```python
from build123d import *

# Parameters (mm, degrees)
SKETCH_1_W          = 20
SKETCH_1_H          = 20
EXTRUDE_1_DEPTH     = 182
SKETCH_3_W          = 35
SKETCH_3_H          = 35
EXTRUDE_2_DEPTH     = 3
SKETCH_4_R          = 2.1
CUT_EXTRUDE_2_DEPTH = 23
CUT_EXTRUDE_3_REACH = 188.648
SKETCH_5_R          = 1.6
EXTRUDE_3_DEPTH     = 20
EXTRUDE_4_DEPTH     = 20
FILLET_1_R          = 2
CUT_EXTRUDE_4_REACH = 186.903
SKETCH_8_W          = 62
SKETCH_8_H          = 12
CUT_EXTRUDE_6_REACH = 186.896


with BuildPart() as part:
    # 草图1 → 凸台-拉伸1 (new body)
    with BuildSketch(Plane(origin=(0, 0, 0), x_dir=(0, 0, -1), z_dir=(1, 0, 0))):
        Rectangle(SKETCH_1_W, SKETCH_1_H)
    extrude(amount=EXTRUDE_1_DEPTH)

    # 草图3 → 凸台-拉伸2 (add)
    with BuildSketch(Plane.ZY):
        Rectangle(SKETCH_3_W, SKETCH_3_H)
    extrude(amount=EXTRUDE_2_DEPTH)

    # 草图4 → 切除-拉伸2 (cut)
    with BuildSketch(Plane(origin=(182, 0, 0), x_dir=(0, 0, -1), z_dir=(1, 0, 0))):
        Circle(SKETCH_4_R)
    extrude(amount=-CUT_EXTRUDE_2_DEPTH, mode=Mode.SUBTRACT)

    # 草图5 → 切除-拉伸3 (cut, up to next)
    with BuildSketch(Plane.ZY.offset(3), mode=Mode.PRIVATE) as cut_extrude_3_sk1:
        with Locations((-14, 14)):
            Circle(SKETCH_5_R)
    cut_extrude_3_tool1 = extrude(cut_extrude_3_sk1.sketch, amount=-CUT_EXTRUDE_3_REACH, mode=Mode.PRIVATE) & part.part
    # 草图5 → 切除-拉伸3 (cut, up to next)
    with BuildSketch(Plane.ZY.offset(3), mode=Mode.PRIVATE) as cut_extrude_3_sk2:
        with Locations((14, 14)):
            Circle(SKETCH_5_R)
    cut_extrude_3_tool2 = extrude(cut_extrude_3_sk2.sketch, amount=-CUT_EXTRUDE_3_REACH, mode=Mode.PRIVATE) & part.part
    # 草图5 → 切除-拉伸3 (cut, up to next)
    with BuildSketch(Plane.ZY.offset(3), mode=Mode.PRIVATE) as cut_extrude_3_sk3:
        with Locations((-14, -14)):
            Circle(SKETCH_5_R)
    cut_extrude_3_tool3 = extrude(cut_extrude_3_sk3.sketch, amount=-CUT_EXTRUDE_3_REACH, mode=Mode.PRIVATE) & part.part
    # 草图5 → 切除-拉伸3 (cut, up to next)
    with BuildSketch(Plane.ZY.offset(3), mode=Mode.PRIVATE) as cut_extrude_3_sk4:
        with Locations((14, -14)):
            Circle(SKETCH_5_R)
    cut_extrude_3_tool4 = extrude(cut_extrude_3_sk4.sketch, amount=-CUT_EXTRUDE_3_REACH, mode=Mode.PRIVATE) & part.part
    add(cut_extrude_3_tool1.solids().sort_by_distance((-3, 14, -14))[0], mode=Mode.SUBTRACT)
    add(cut_extrude_3_tool2.solids().sort_by_distance((-3, 14, 14))[0], mode=Mode.SUBTRACT)
    add(cut_extrude_3_tool3.solids().sort_by_distance((-3, -14, -14))[0], mode=Mode.SUBTRACT)
    add(cut_extrude_3_tool4.solids().sort_by_distance((-3, -14, 14))[0], mode=Mode.SUBTRACT)

    # 草图6 → 凸台-拉伸3 (add)
    with BuildSketch(Plane(origin=(0, 0, -10), x_dir=(-1, 0, 0), z_dir=(0, 0, -1))):
        Polygon((-30, 10), (0, 17.5), (0, 10), align=None)
        Polygon((0, -10), (-30, -10), (0, -17.5), align=None)
    extrude(amount=-EXTRUDE_3_DEPTH)

    # 草图7 → 凸台-拉伸4 (add)
    with BuildSketch(Plane(origin=(0, 10, 0), x_dir=(1, 0, 0), z_dir=(0, 1, 0))):
        Polygon((0, 10), (30, 10), (0, 17.5), align=None)
        Polygon((30, -10), (0, -10), (0, -17.550639808), align=None)
    extrude(amount=-EXTRUDE_4_DEPTH)

    # 圆角1
    # the kernel refuses this fillet: 2 mm, written as the material it adds along each edge
    with BuildSketch(Plane(origin=(-5, 10, -10), x_dir=(0, 0, -1), z_dir=(1, 0, 0))) as fillet_1_piece_1_section:
        with BuildLine():
            CenterArc((FILLET_1_R, FILLET_1_R), FILLET_1_R, 180, 90)
            Line((0, FILLET_1_R), (0, 0))
            Line((0, 0), (FILLET_1_R, 0))
        make_face()
    fillet_1_piece_1 = extrude(amount=40, mode=Mode.PRIVATE)
    fillet_1_piece_1 = split(fillet_1_piece_1, bisect_by=Plane(origin=(14.470095562, 13.882476109, -10.438694278), z_dir=(-0.24253562503633314, -0.9701425001453319, 0)), keep=Keep.TOP, mode=Mode.PRIVATE)
    fillet_1_piece_1 = split(fillet_1_piece_1, bisect_by=Plane(origin=(-3, 10.438694278, -10.438694278), z_dir=(1, 0, 0)), keep=Keep.TOP, mode=Mode.PRIVATE)
    fillet_1_piece_1 = split(fillet_1_piece_1, bisect_by=Plane(origin=(14.470095562, 10.438694278, -13.882476109), z_dir=(-0.24253562503633308, 0, 0.9701425001453319)), keep=Keep.TOP, mode=Mode.PRIVATE)
    add(fillet_1_piece_1)
    with BuildSketch(Plane(origin=(0, -10, -10), x_dir=(0, -1, 0), z_dir=(1, 0, 0))) as fillet_1_piece_2_section:
        with BuildLine():
            CenterArc((FILLET_1_R, FILLET_1_R), FILLET_1_R, 180, 90)
            Line((0, FILLET_1_R), (0, 0))
            Line((0, 0), (FILLET_1_R, 0))
        make_face()
    fillet_1_piece_2 = extrude(amount=35, mode=Mode.PRIVATE)
    fillet_1_piece_2 = split(fillet_1_piece_2, bisect_by=Plane(origin=(14.470095562, -10.438694278, -13.882476109), z_dir=(-0.24253562503633308, 0, 0.9701425001453319)), keep=Keep.TOP, mode=Mode.PRIVATE)
    fillet_1_piece_2 = split(fillet_1_piece_2, bisect_by=Plane(origin=(14.470095562, -13.882476109, -10.438694278), z_dir=(-0.24253562503633314, 0.9701425001453319, 0)), keep=Keep.TOP, mode=Mode.PRIVATE)
    add(fillet_1_piece_2)
    with BuildSketch(Plane(origin=(35, 10, 10), x_dir=(0, 1, 0), z_dir=(-1, 0, 0))) as fillet_1_piece_3_section:
        with BuildLine():
            CenterArc((FILLET_1_R, -FILLET_1_R), FILLET_1_R, 90, 90)
            Line((0, -FILLET_1_R), (0, 0))
            Line((0, 0), (FILLET_1_R, 0))
        make_face()
    fillet_1_piece_3 = extrude(amount=40, mode=Mode.PRIVATE)
    fillet_1_piece_3 = split(fillet_1_piece_3, bisect_by=Plane(origin=(14.474382617, 13.881404346, 10.438850692), z_dir=(-0.24253562503633314, -0.9701425001453319, 0)), keep=Keep.TOP, mode=Mode.PRIVATE)
    fillet_1_piece_3 = split(fillet_1_piece_3, bisect_by=Plane(origin=(-3, 10.438597443, 10.438850692), z_dir=(1, 0, 0)), keep=Keep.TOP, mode=Mode.PRIVATE)
    fillet_1_piece_3 = split(fillet_1_piece_3, bisect_by=Plane(origin=(14.485990983, 10.438597443, 13.904689802), z_dir=(-0.24407597060240918, 0, -0.969756113966028)), keep=Keep.TOP, mode=Mode.PRIVATE)
    add(fillet_1_piece_3)
    with BuildSketch(Plane(origin=(35, -10, 10), x_dir=(0, 0, 1), z_dir=(-1, 0, 0))) as fillet_1_piece_4_section:
        with BuildLine():
            CenterArc((FILLET_1_R, -FILLET_1_R), FILLET_1_R, 90, 90)
            Line((0, -FILLET_1_R), (0, 0))
            Line((0, 0), (FILLET_1_R, 0))
        make_face()
    fillet_1_piece_4 = extrude(amount=35, mode=Mode.PRIVATE)
    fillet_1_piece_4 = split(fillet_1_piece_4, bisect_by=Plane(origin=(14.474382617, -13.881404346, 10.438850692), z_dir=(-0.24253562503633314, 0.9701425001453319, 0)), keep=Keep.TOP, mode=Mode.PRIVATE)
    fillet_1_piece_4 = split(fillet_1_piece_4, bisect_by=Plane(origin=(14.485990983, -10.438597443, 13.904689802), z_dir=(-0.24407597060240918, 0, -0.969756113966028)), keep=Keep.TOP, mode=Mode.PRIVATE)
    add(fillet_1_piece_4)

    # 草图8 → 切除-拉伸4 (cut, up to next)
    with BuildSketch(Plane(origin=(0, 0, -10), x_dir=(-1, 0, 0), z_dir=(0, 0, -1)), mode=Mode.PRIVATE) as cut_extrude_4_sk1:
        with Locations((-147, 0)):
            Rectangle(SKETCH_8_W, SKETCH_8_H)
    cut_extrude_4_tool1 = extrude(cut_extrude_4_sk1.sketch, amount=-CUT_EXTRUDE_4_REACH, mode=Mode.PRIVATE) & part.part
    add(cut_extrude_4_tool1.solids().sort_by_distance((147, 0, -10))[0], mode=Mode.SUBTRACT)

    # 草图9 → 切除-拉伸6 (cut, up to next)
    with BuildSketch(Plane.XY.offset(10), mode=Mode.PRIVATE) as cut_extrude_6_sk1:
        with BuildLine():
            Line((97.964235065, 6.297490727), (107.103469291, -2.781172596))
            ThreePointArc((107.103469291, -2.781172596), (107.115824812, -6.497340056), (103.399657352, -6.509695577))
            Line((103.399657352, -6.509695577), (94.260423126, 2.568967746))
            ThreePointArc((94.260423126, 2.568967746), (94.248067605, 6.285135206), (97.964235065, 6.297490727))
        make_face()
    cut_extrude_6_tool1 = extrude(cut_extrude_6_sk1.sketch, amount=-CUT_EXTRUDE_6_REACH, mode=Mode.PRIVATE) & part.part
    # 草图9 → 切除-拉伸6 (cut, up to next)
    with BuildSketch(Plane.XY.offset(10), mode=Mode.PRIVATE) as cut_extrude_6_sk2:
        with BuildLine():
            Line((82.964235065, 6.297490727), (92.103469291, -2.781172596))
            ThreePointArc((92.103469291, -2.781172596), (92.115824812, -6.497340056), (88.399657352, -6.509695577))
            Line((88.399657352, -6.509695577), (79.260423126, 2.568967746))
            ThreePointArc((79.260423126, 2.568967746), (79.248067605, 6.285135206), (82.964235065, 6.297490727))
        make_face()
    cut_extrude_6_tool2 = extrude(cut_extrude_6_sk2.sketch, amount=-CUT_EXTRUDE_6_REACH, mode=Mode.PRIVATE) & part.part
    # 草图9 → 切除-拉伸6 (cut, up to next)
    with BuildSketch(Plane.XY.offset(10), mode=Mode.PRIVATE) as cut_extrude_6_sk3:
        with BuildLine():
            Line((67.964235065, 6.297490727), (77.103469291, -2.781172596))
            ThreePointArc((77.103469291, -2.781172596), (77.115824812, -6.497340056), (73.399657352, -6.509695577))
            Line((73.399657352, -6.509695577), (64.260423126, 2.568967746))
            ThreePointArc((64.260423126, 2.568967746), (64.248067605, 6.285135206), (67.964235065, 6.297490727))
        make_face()
    cut_extrude_6_tool3 = extrude(cut_extrude_6_sk3.sketch, amount=-CUT_EXTRUDE_6_REACH, mode=Mode.PRIVATE) & part.part
    # 草图9 → 切除-拉伸6 (cut, up to next)
    with BuildSketch(Plane.XY.offset(10), mode=Mode.PRIVATE) as cut_extrude_6_sk4:
        with BuildLine():
            Line((52.964235065, 6.297490727), (62.103469291, -2.781172596))
            ThreePointArc((62.103469291, -2.781172596), (62.115824812, -6.497340056), (58.399657352, -6.509695577))
            Line((58.399657352, -6.509695577), (49.260423126, 2.568967746))
            ThreePointArc((49.260423126, 2.568967746), (49.248067605, 6.285135206), (52.964235065, 6.297490727))
        make_face()
    cut_extrude_6_tool4 = extrude(cut_extrude_6_sk4.sketch, amount=-CUT_EXTRUDE_6_REACH, mode=Mode.PRIVATE) & part.part
    # 草图9 → 切除-拉伸6 (cut, up to next)
    with BuildSketch(Plane.XY.offset(10), mode=Mode.PRIVATE) as cut_extrude_6_sk5:
        with BuildLine():
            Line((37.964235065, 6.297490727), (47.103469291, -2.781172596))
            ThreePointArc((47.103469291, -2.781172596), (47.115824812, -6.497340056), (43.399657352, -6.509695577))
            Line((43.399657352, -6.509695577), (34.260423126, 2.568967746))
            ThreePointArc((34.260423126, 2.568967746), (34.248067605, 6.285135206), (37.964235065, 6.297490727))
        make_face()
    cut_extrude_6_tool5 = extrude(cut_extrude_6_sk5.sketch, amount=-CUT_EXTRUDE_6_REACH, mode=Mode.PRIVATE) & part.part
    add(cut_extrude_6_tool1.solids().sort_by_distance((100.681946, -0.106102, 10))[0], mode=Mode.SUBTRACT)
    add(cut_extrude_6_tool2.solids().sort_by_distance((85.681946, -0.106102, 10))[0], mode=Mode.SUBTRACT)
    add(cut_extrude_6_tool3.solids().sort_by_distance((70.681946, -0.106102, 10))[0], mode=Mode.SUBTRACT)
    add(cut_extrude_6_tool4.solids().sort_by_distance((55.681946, -0.106102, 10))[0], mode=Mode.SUBTRACT)
    add(cut_extrude_6_tool5.solids().sort_by_distance((40.681946, -0.106102, 10))[0], mode=Mode.SUBTRACT)


solid = part.part
```
Can you work these out from the model? Positions are in its coordinate system, mm. A direction names the side the tool comes from. Round coordinates to 2 decimals unless told otherwise and drop trailing zeros. Loops run counter-clockwise (first coordinate to the right, second up) from the corner with the lowest first, then second, coordinate; pieces in that order, holes last.
Item 1: Will these pins go through, and if not, where does the flat tip stop? pin 1 Ø1.5 at (x, z) = (157, -2.5) entering from -Y; pin 2 Ø4.5 at (x, z) = (10.5, -14) entering from +Y; pin 3 Ø5 at (x, y) = (65.5, 0.5) entering from +Z.
Item 2: Suppose I cut it at A-A, the plane x = 150. Write out the boundary of the cut face in (y, z), then the cut area to 3 significant figures.
Item 3: Suppose I cut it at C-C, the plane z = -5.5. State how many separate pieces and enclosed holes the cut face has, then the cut area to 3 significant figures.
Item 4: Suppose I cut it at B-B, the plane y = -14. Write out the boundary of the cut face in (x, z), then the cut area to 3 significant figures.
Item 5: Suppose I cut it at D-D, the plane z = 14. Write out the boundary of the cut face in (x, y).
Item 6: Which directions (+Z, -Z, +X, -X, +Y, -Y) give clear straight access to the entire face, cutting with the end or side of a thin tool? Please do faces 1 (the flat face through (0, 14, 12)), 2 (the flat face through (53.89, -2.03, 0.14)), 3 (the flat face through (0, -12, -14)).
Item 7: If we mould it in two halves opening along Y, with no side actions, what happens to faces 4 (the flat face through (8, -14, 10)), 5 (the flat face through (102.47, 1.82, 0.14)), 6 (the flat face through (105, 10, 0))? For each: +Y half, -Y half, draft (parallel to the pull), parting line (faces both ways), or undercut.
Item 8: Please list where these lines run through material, in increasing order: L1, parallel to Y at x = -1, z = -14; L2, parallel to Y at x = 142, z = 5.5; L3, parallel to Y at x = 179.05, z = 0.
Reported:
1. pin 1: stops at y = -10
1. pin 2: stops at y = 10.02
1. pin 3: stops at z = 10
2. outline: (-10, -10) - (-6, -10) - (-6, 10) - (-10, 10) - close; (6, -10) - (10, -10) - (10, 10) - (6, 10) - close
2. area: 160 mm2
3. separate pieces: 1
3. enclosed holes: 6
3. area: 2,780 mm2
4. outline: (-3, -17.5) - (0, -17.5) - (0, -15.6) - (-3, -15.6) - close; (-3, -12.4) - (0, -12.4) - (0, -10) - (14, -10) - (14, 10) - (0, 10) - (0, 12.4) - (-3, 12.4) - close; (-3, 15.6) - (0, 15.6) - (0, 17.5) - (-3, 17.5) - close
4. area: 366 mm2
5. outline: (-3, -17.5) - (0, -17.5) - (0, -15.6) - (-3, -15.6) - close; (-3, -12.4) - (0, -12.4) - (0, -10) - (14.11, -10) - (14.11, 10) - (0, 10) - (0, 12.4) - (-3, 12.4) - close; (-3, 15.6) - (0, 15.6) - (0, 17.5) - (-3, 17.5) - close
6. face 1: +Z, +X, +Y
6. face 2: +Z, -Z
6. face 3: -Z, +X, -Y
7. face 4: draft
7. face 5: undercut
7. face 6: +Y half
8. L1: y = -17.5 to -15.6, -12.4 to 12.4, 15.6 to 17.5
8. L2: y = -10 to -6, 6 to 10
8. L3: y = -10 to -2.1, 2.1 to 10
